```python
from build123d import *

# Parameters (mm, degrees)
SKETCH1_R           = 3.175
SKETCH1_W           = 4.7625
SKETCH1_H           = 25.4
BOSS_EXTRUDE1_DEPTH = 4.7625


with BuildPart() as part:
    # Sketch1 → Boss-Extrude1 (new body)
    with BuildSketch(Plane.XY):
        Polygon((80.9625, 0), (127, 0), (127, 177.8), (0, 177.8), (0, 0), (76.2, 0), (76.2, 25.4), (80.9625, 25.4), align=None)
        with Locations((120.65, 171.45)):
            Circle(SKETCH1_R, mode=Mode.SUBTRACT)
        with Locations((78.58125, 139.7)):
            Rectangle(SKETCH1_W, SKETCH1_H, mode=Mode.SUBTRACT)
        with BuildLine():
            ThreePointArc((10.07830682, 171.45), (20.074522157, 130.072156721), (44.202038564, 95.002038564))
            ThreePointArc((44.202038564, 95.002038564), (48.153351257, 95.002038564), (48.153351257, 98.953351257))
            ThreePointArc((48.153351257, 98.953351257), (25.239205738, 132.21130856), (15.674955486, 171.45))
            ThreePointArc((15.674955486, 171.45), (12.876631153, 174.248324333), (10.07830682, 171.45))
        make_face(mode=Mode.SUBTRACT)
    extrude(amount=BOSS_EXTRUDE1_DEPTH)


solid = part.part
```
Input: part model. Units: mm. Frame: model coordinates. A direction names the side the tool comes from. Give positions to 0.01 mm unless a question says otherwise; leave off trailing zeros. Order: outer loops, then holes, each group sorted by start corner. A loop starts at its lowest first (then second) coordinate and runs counter-clockwise, first axis right, second up. Notation, with made-up numbers: M -33,35.25 L 6,35.25 A15 cw 6,59.25 Z; hole C 28,-15.75 d6. An arc over 180 degrees is marked long. One line per question, with ' | ' between items.
1) Draft query along X for faces 4 (the face through (63, 90, 0)), 5 (the face through (12.938, 174.248, 2.348)), 6 (the face through (127, 88, 2)). Return one class per face: pulls with the +X half, pulls with the -X half, needs draft (parallel to the pull), parting line crosses it, or undercut.
Filled in:
face 4: needs draft | face 5: undercut | face 6: pulls with the +X half
2) Contact query for flat-ended pins moving along their axis: P1, Ø7.5, axis at x = 120.65, y = 171.45, coming from the +Z side; P2, Ø1.4, axis at x = 79, z = 3, coming from the -Y side. Output: stop coordinate, or through.
Filled in:
P1: stops at z = 4.76 | P2: stops at y = 25.4
3) Section B-B on x = 120.65. Output: boundary loops of the cut face in (y, z) (1 decimal), and give its area (3 significant figures).
Filled in:
outline: M 0,0 L 168.3,0 L 168.3,4.8 L 0,4.8 Z; M 174.6,0 L 177.8,0 L 177.8,4.8 L 174.6,4.8 Z | area: 817 mm2
4) Access query for faces 1 (the face through (64, 177.8, 2)), 2 (the face through (79, 152.4, 2)), 3 (the face through (76.2, 13, 2)). Directions: +Z, -Z, +X, -X, +Y, -Y. A direction counts if a zero-diameter tool reaches every point of the face in a straight line with its end or side. Return the directions, or none.
Filled in:
face 1: +Z, -Z, +X, -X, +Y | face 2: +Z, -Z | face 3: +Z, -Z, -Y
5) Section C-C on y = 136. Output: boundary loops of the cut face in (x, z), and give its area (3 significant figures).
Filled in:
outline: M 0,0 L 17.62,0 L 17.62,4.76 L 0,4.76 Z; M 23.63,0 L 76.2,0 L 76.2,4.76 L 23.63,4.76 Z; M 80.96,0 L 127,0 L 127,4.76 L 80.96,4.76 Z | area: 554 mm2
6) Section D-D on y = 111. Output: boundary loops of the cut face in (x, z).
Filled in:
outline: M 0,0 L 30.83,0 L 30.83,4.76 L 0,4.76 Z; M 37.72,0 L 127,0 L 127,4.76 L 37.72,4.76 Z
7) Ray query, L1, parallel to X at y = 171.45, z = 1.7 (3 decimals); L2, parallel to Y at x = 80.5, z = 1.3; L3, parallel to X at y = 151, z = 2.75. Return the intervals inside material, ascending.
Filled in:
L1: x = 0 to 10.078, 15.675 to 117.475, 123.825 to 127 | L2: y = 25.4 to 127, 152.4 to 177.8 | L3: x = 0 to 13.01, 18.76 to 76.2, 80.96 to 127
8) Section A-A on z = 3.85. State how many separate pieces and enclosed holes the cut face has, and give its area (3 significant figures).
Filled in:
separate pieces: 1 | enclosed holes: 3 | area: 21,800 mm2
